from build123d import *

# Parameters (mm, degrees)
EXTRUDE_1_DEPTH      = 2
EXTRUDE_1_DEPTH_BACK = 7
SKETCH_1_R           = 6.5
SKETCH_1_R_2         = 3
CHAMFER_1_SIZE       = 1
CHAMFER_2_SIZE       = 0.5


with BuildPart() as part:
    # Эскиз1 → Бобышка-Вытянуть1 (new, two sides: drawn at the far end of the back side and taken through both)
    with BuildSketch(Plane.XY.offset(-EXTRUDE_1_DEPTH_BACK)):
        with Locations((135, 20)):
            Circle(SKETCH_1_R)
        with Locations((135, 20)):
            Circle(SKETCH_1_R_2, mode=Mode.SUBTRACT)
    extrude(amount=EXTRUDE_1_DEPTH + EXTRUDE_1_DEPTH_BACK)

    # Фаска1
    chamfer_1_edges = [part.edges().sort_by_distance(p)[0] for p in [
        (132, 20, 2),
    ]]
    chamfer(chamfer_1_edges, length=CHAMFER_1_SIZE)

    # Фаска2
    chamfer_2_edges = [part.edges().sort_by_distance(p)[0] for p in [
        (128.5, 20, 2),
    ]]
    chamfer(chamfer_2_edges, length=CHAMFER_2_SIZE)


solid = part.part
Could you check a few things on this model? Use its own coordinates, in mm. Round coordinates to 2 decimals unless told otherwise and drop trailing zeros. Write each loop counter-clockwise with the first axis right and the second up, starting at its lowest first coordinate (ties: lowest second). Pieces come first, ordered by that corner, then holes. Notation, with made-up numbers: (-22.5, 3) -> (17.5, 3) arc R10 ccw to (17.5, 21) -> close; hole circle Ø8 at (-5, 7). An arc over 180 degrees is marked (long way). Use a Markdown table: item, result.
1. If we section it at A-A (y = 20): List the corners of the cut face in (x, z) for me, then the cut area to 4 significant figures.
Answer key:
| item | result |
|---|---|
| outline | (128.5, -7) -> (132, -7) -> (132, 1) -> (131, 2) -> (129, 2) -> (128.5, 1.5) -> close; (138, -7) -> (141.5, -7) -> (141.5, 1.5) -> (141, 2) -> (139, 2) -> (138, 1) -> close |
| area | 61.75 mm^2 |
2. If we section it at C-C (z = 0): List the corners of the cut face in (x, y) for me, then the cut area to 3 significant figures.
Answer key:
| item | result |
|---|---|
| outline | circle Ø13 at (135, 20); hole circle Ø6 at (135, 20) |
| area | 104 mm^2 |
3. If we section it at B-B (x = 135): List the corners of the cut face in (y, z) for me, then the cut area to 4 significant figures.
Answer key:
| item | result |
|---|---|
| outline | (13.5, -7) -> (17, -7) -> (17, 1) -> (16, 2) -> (14, 2) -> (13.5, 1.5) -> close; (23, -7) -> (26.5, -7) -> (26.5, 1.5) -> (26, 2) -> (24, 2) -> (23, 1) -> close |
| area | 61.75 mm^2 |
4. Please list where these lines run through material, in increasing order: probe 1 along Y at (x, z) = (135, -2); probe 2 along Y at (x, z) = (136, -5.5); probe 3 along X at (y, z) = (20.5, 0).
Answer key:
| item | result |
|---|---|
| probe 1 | y = 13.5 to 17, 23 to 26.5 |
| probe 2 | y = 13.58 to 17.17, 22.83 to 26.42 |
| probe 3 | x = 128.52 to 132.04, 137.96 to 141.48 |
5. We'd pull the mould along Y, two halves only. Please class faces 1 (the face through (128.506, 20.286, -2.81)), 2 (the face through (138, 19, -7)), 3 (the face through (137.86, 20.9, -3.06)): +Y half, -Y half, draft (parallel to the pull), parting line (faces both ways), or undercut.
Answer key:
| item | result |
|---|---|
| face 1 | parting line |
| face 2 | draft |
| face 3 | undercut |
6. For pin 1 Ø1 at (x, z) = (131.5, -3.5) entering from -Y; pin 2 Ø1.5 at (y, z) = (21, -1.5) entering from -X; pin 3 Ø6 at (x, y) = (135.5, 20.5) entering from +Z, each with a flat end and sliding along its axis, tell me the tip position at first contact or that it passes through.
Answer key:
| item | result |
|---|---|
| pin 1 | stops at y = 14.23 |
| pin 2 | stops at x = 128.5 |
| pin 3 | stops at z = 1.71 |
